Part model, mm, in its own coordinate system. Round coordinates to 2 decimals unless told otherwise and drop trailing zeros. Order: outer loops, then holes, each group sorted by start corner. A loop starts at its lowest first (then second) coordinate and runs counter-clockwise, first axis right, second up. Notation, with made-up numbers: (39.25, -33) - (45.25, -33) arc R28 ccw to (45.25, -13) - close; hole circle Ø10 at (19, 40.5). An arc over 180 degrees is marked (long way). Return JSON: item names as keys, results as strings. Group by question number.
Item 1: Saw through at D-D on z = 3.5. List the corners of the cut face in (x, y), and give its area (3 significant figures).
Item 2: Probe probe 1 along X at (y, z) = (-0.6, 0); probe 2 along Z at (x, y) = (1.5, 1); probe 3 along Z at (x, y) = (53, 0.65). List the from-to ranges inside material, lowest first.
Item 3: Saw through at A-A on z = 0. List the corners of the cut face in (x, y), and give its area (3 significant figures).
Item 4: Saw through at B-B on y = -0.15. List the corners of the cut face in (x, z), and give its area (3 significant figures).
Item 5: Drop flat-ended pins along their axis: pin 1 (1.2 mm diameter, centred on y = 0, z = -0.5, fed in from -X); pin 2 (1.5 mm diameter, centred on y = 0.5, z = 6.5, fed in from +X). Give the stop position or say it passes through.
Item 6: Saw through at C-C on x = 46.5. List the corners of the cut face in (y, z), and give its area (3 significant figures).
```python
from build123d import *

# Parameters (mm, degrees)
SKETCH1_R           = 5
BOSS_EXTRUDE1_DEPTH = 1.5


with BuildPart() as part:
    # Sketch1 → Boss-Extrude1 (new, symmetric)
    with BuildSketch(Plane(origin=(0, 0, 0), x_dir=(1, 0, 0), z_dir=(0, 1, 0))):
        with BuildLine():
            Line((50, 9), (0, 9))
            ThreePointArc((0, 9), (-9, 0), (0, -9))
            Line((0, -9), (50, -9))
            ThreePointArc((50, -9), (59, 0), (50, 9))
        make_face()
        with BuildLine():
            ThreePointArc((4.841229183, -1.25), (-5, 0), (4.841229183, 1.25))
            Line((4.841229183, 1.25), (7, 1.25))
            Line((7, 1.25), (7, -1.25))
            Line((7, -1.25), (4.841229183, -1.25))
        make_face(mode=Mode.SUBTRACT)
        with Locations(Location((50, 0, 0), (0, 0, 270))):
            Circle(SKETCH1_R, mode=Mode.SUBTRACT)
    extrude(amount=BOSS_EXTRUDE1_DEPTH, both=True)


solid = part.part
```
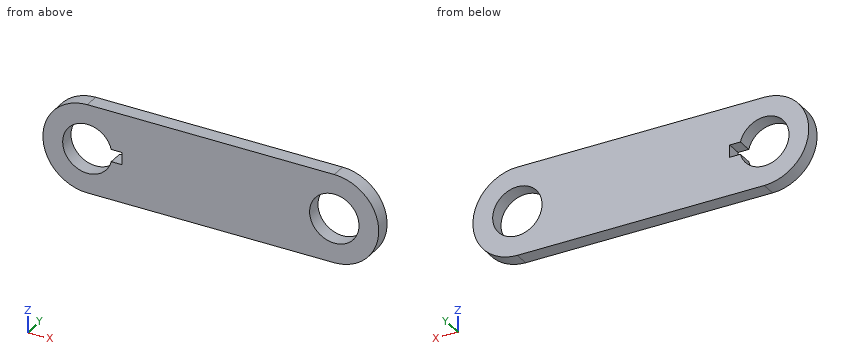
Filled in:
{
 "1": {"outline": "(-8.29, -1.5) - (-3.57, -1.5) - (-3.57, 1.5) - (-8.29, 1.5) - close; (3.57, -1.5) - (46.43, -1.5) - (46.43, 1.5) - (3.57, 1.5) - close; (53.57, -1.5) - (58.29, -1.5) - (58.29, 1.5) - (53.57, 1.5) - close", "area": "157 mm^2"},
 "2": {"probe 1": "x = -9 to -5, 7 to 45, 55 to 59", "probe 2": "z = -9 to -4.77, 4.77 to 9", "probe 3": "z = -8.49 to -4, 4 to 8.49"},
 "3": {"outline": "(-9, -1.5) - (-5, -1.5) - (-5, 1.5) - (-9, 1.5) - close; (7, -1.5) - (45, -1.5) - (45, 1.5) - (7, 1.5) - close; (55, -1.5) - (59, -1.5) - (59, 1.5) - (55, 1.5) - close", "area": "138 mm^2"},
 "4": {"outline": "(0, -9) - (50, -9) arc R9 ccw to (50, 9) - (0, 9) arc R9 ccw to start; hole (4.84, -1.25) - (7, -1.25) - (7, 1.25) - (4.84, 1.25) arc R5 ccw (long way) to start; hole circle Ø10 at (50, 0)", "area": "992 mm^2"},
 "5": {"pin 1": "stops at x = -9", "pin 2": "stops at x = 56.92"},
 "6": {"outline": "(-1.5, -9) - (1.5, -9) - (1.5, -3.57) - (-1.5, -3.57) - close; (-1.5, 3.57) - (1.5, 3.57) - (1.5, 9) - (-1.5, 9) - close", "area": "32.6 mm^2"}
}
